Here's how the part is built. I have some questions about the finished solid (model axes, mm). A direction names the side the tool comes from. Coordinates: 2 decimals unless noted, no trailing zeros. Write each loop counter-clockwise with the first axis right and the second up, starting at its lowest first coordinate (ties: lowest second). Pieces come first, ordered by that corner, then holes.
Item 1: I want a section at D-D (y = -7). Please give me the cut outline in (x, z), and give its area (3 significant figures).
Item 2: Please list where these lines run through material, in increasing order: line 1 (Z direction, x = -5.5, y = 29.5); line 2 (Z direction, x = -20.5, y = -33.5); line 3 (Z direction, x = -24.5, y = 21).
Item 3: For faces 1 (the face through (20, -7, 95)), 2 (the face through (-14, 41, 37)), 3 (the face through (-6.92, -3.49, 107.6)), 4 (the face through (-5, 44, 110)), 5 (the face through (0, 58, 18)), which set-ups out of +Z, -Z, +X, -X, +Y, -Y let a thin tool reach every point of the face, with its end or its side?
Item 4: I want a section at B-B (x = 20). Please give me the cut outline in (y, z), and give its area (3 significant figures).
Item 5: If we mould it in two halves opening along X, with no side actions, what happens to faces 6 (the face through (5, 43, 13)), 7 (the face through (20, -7, 5)), 8 (the face through (2, 36, 3))? For each: pulls with the +X half, pulls with the -X half, needs draft (parallel to the pull), parting line crosses it, or undercut.
Item 6: I want a section at A-A (z = 27). Please give me the cut outline in (x, y), and give its area (3 significant figures).
Item 7: I'm going to push flat-ended pins straight in: P1, Ø2, axis at x = -6, z = 25.5, coming from the -Y side; P2, Ø16.5, axis at y = 46, z = 93.5, coming from the +X side; P3, Ø5, axis at x = 19, z = 15, coming from the +Y side; P4, Ø4.5, axis at y = 57.5, z = 9.5, coming from the +X side. Where does each tip first touch, or does it pass through?
Item 8: I want a section at C-C (z = 66.5). Please give me the cut outline in (x, y).
from build123d import *

# Parameters (mm, degrees)
BOSS_EXTRUDE1_DEPTH      = 115
CUT_EXTRUDE1_DEPTH       = 15
SKETCH3_W                = 21
SKETCH3_H                = 15
BOSS_EXTRUDE2_DEPTH      = 10
BOSS_EXTRUDE2_DEPTH_BACK = 110
SKETCH4_W                = 33
SKETCH4_H                = 40
CUT_EXTRUDE2_DEPTH       = 31
CUT_EXTRUDE2_DEPTH_BACK  = 46.5
CUT_EXTRUDE3_DEPTH       = 67
CUT_EXTRUDE3_DEPTH_BACK  = 41.362796982
FILLET1_R                = 10


with BuildPart() as part:
    # Sketch1 → Boss-Extrude1 (new body)
    with BuildSketch(Plane.XY):
        with BuildLine():
            Line((0, 0), (0, 66))
            ThreePointArc((0, 66), (-45.256322222, 16.603413808), (-10, -40.362796982))
            Line((-10, -40.362796982), (-10, -15))
            Line((-10, -15), (30, -15))
            Line((30, -15), (30, 0))
            Line((30, 0), (0, 0))
        make_face()
    extrude(amount=BOSS_EXTRUDE1_DEPTH)

    # Sketch2 → Cut-Extrude1 (cut)
    with BuildSketch(Plane.XY.offset(115)):
        with BuildLine():
            Line((30, -10), (-44.890423857, 3.205202323))
            ThreePointArc((-44.890423857, 3.205202323), (-35.149622711, 43.684665376), (0, 66))
            Line((0, 66), (0, 0))
            Line((0, 0), (30, 0))
            Line((30, 0), (30, -10))
        make_face()
    extrude(amount=-CUT_EXTRUDE1_DEPTH, mode=Mode.SUBTRACT)

    # Sketch3 → Boss-Extrude2 (add, two sides)
    with BuildSketch(Plane(origin=(0, 0, 0), x_dir=(-1, 0, 0), z_dir=(0, 0, -1))) as boss_extrude2_sk:
        with Locations((5.5, 43.5)):
            Rectangle(SKETCH3_W, SKETCH3_H)
    extrude(amount=BOSS_EXTRUDE2_DEPTH)
    extrude(boss_extrude2_sk.sketch, amount=-BOSS_EXTRUDE2_DEPTH_BACK)

    # Sketch4 → Cut-Extrude2 (cut, two sides)
    with BuildSketch(Plane(origin=(0, 0, 0), x_dir=(0, 0, -1), z_dir=(1, 0, 0))) as cut_extrude2_sk:
        with Locations((-53.5, 46)):
            Rectangle(SKETCH4_W, SKETCH4_H)
    extrude(amount=CUT_EXTRUDE2_DEPTH, mode=Mode.SUBTRACT)
    extrude(cut_extrude2_sk.sketch, amount=-CUT_EXTRUDE2_DEPTH_BACK, mode=Mode.SUBTRACT)

    # Sketch5 → Cut-Extrude3 (cut, two sides)
    with BuildSketch(Plane(origin=(0, 0, 0), x_dir=(1, 0, 0), z_dir=(0, 1, 0))) as cut_extrude3_sk:
        with BuildLine():
            Line((25, -10), (25, -90))
            ThreePointArc((25, -90), (20, -95), (15, -90))
            Line((15, -90), (15, -10))
            ThreePointArc((15, -10), (20, -5), (25, -10))
        make_face()
    extrude(amount=CUT_EXTRUDE3_DEPTH, mode=Mode.SUBTRACT)
    extrude(cut_extrude3_sk.sketch, amount=-CUT_EXTRUDE3_DEPTH_BACK, mode=Mode.SUBTRACT)

    # Fillet1
    fillet1_edges = [part.edges().sort_by_distance(p)[0] for p in [
        (0, 0, 50),
    ]]
    fillet(fillet1_edges, radius=FILLET1_R)


solid = part.part
Answer:
1. outline: (-42.36, 0) - (30, 0) - (30, 100) - (12.99, 100) - (12.99, 115) - (-42.36, 115) - close; hole (15, 10) arc R5 ccw to (25, 10) - (25, 90) arc R5 ccw to (15, 90) - close
1. area: 7,190 mm2
2. line 1: z = 0 to 37, 70 to 100
2. line 2: z = 0 to 115
2. line 3: z = 0 to 100
3. face 1: +Y, -Y
3. face 2: +X, -X, +Y
3. face 3: +Z, +X
3. face 4: +Z, +X, -X, +Y
3. face 5: +Z, -Z, +X, +Y
4. outline: (-15, 0) - (0, 0) - (0, 5) - (-15, 5) - close; (-15, 95) - (0, 95) - (0, 100) - (-8.24, 100) - (-8.24, 115) - (-15, 115) - close
4. area: 251 mm2
5. face 6: pulls with the +X half
5. face 7: undercut
5. face 8: needs draft
6. outline: (-10, -40.36) - (-10, -15) - (15, -15) - (15, 0) - (10, 0) arc R10 cw to (0, 10) - (0, 36) - (5, 36) - (5, 51) - (0, 51) - (0, 66) arc R55.5 ccw to start; (25, -15) - (30, -15) - (30, 0) - (25, 0) - close
6. area: 3,860 mm2
7. P1: stops at y = -15
7. P2: stops at x = 5
7. P3: passes through
7. P4: stops at x = 0
8. outline: (-43.55, 26) arc R55.5 ccw to (-10, -40.36) - (-10, -15) - (15, -15) - (15, 0) - (10, 0) arc R10 cw to (0, 10) - (0, 26) - close; (25, -15) - (30, -15) - (30, 0) - (25, 0) - close
